Input: part model. Units: mm. Frame: model coordinates. A direction names the side the tool comes from. Give positions to 0.01 mm unless a question says otherwise; leave off trailing zeros. Loops run counter-clockwise (first coordinate to the right, second up) from the corner with the lowest first, then second, coordinate; pieces in that order, holes last. Notation, with made-up numbers: (-37, 35) - (-21, 35) arc R35 cw to (-21, 72) - close; hole circle Ø3 at (8, 47.5). An arc over 180 degrees is marked (long way). One line per item, written item: value.
from build123d import *

# Parameters (mm, degrees)
F0_W     = 40
F0_H     = 16
F1_DEPTH = 9.6
F2_R     = 2.4
F3_DEPTH = 1.8
F4_T     = -1.8


with BuildPart() as f1:
    # F0 (on Top) → F1 (new body)
    with BuildSketch(Plane.XY):
        with Locations((-20, 8)):
            Rectangle(F0_W, F0_H)
    extrude(amount=F1_DEPTH)

    # F2 (on face) → F3 (join)
    with BuildSketch(Plane.XY.offset(9.6)):
        with Locations((-36, 12)):
            Circle(F2_R)
        with Locations((-36, 4)):
            Circle(F2_R)
        with Locations((-28, 4)):
            Circle(F2_R)
        with Locations((-28, 12)):
            Circle(F2_R)
        with Locations((-20, 4)):
            Circle(F2_R)
        with Locations((-12, 4)):
            Circle(F2_R)
        with Locations((-4, 4)):
            Circle(F2_R)
        with Locations((-4, 12)):
            Circle(F2_R)
        with Locations((-12, 12)):
            Circle(F2_R)
        with Locations((-20, 12)):
            Circle(F2_R)
    extrude(amount=F3_DEPTH)

    # F4
    f4_openings = [f1.faces().sort_by_distance(p)[0] for p in [
        (-20, 8, 0),
    ]]
    offset(amount=F4_T, openings=f4_openings, kind=Kind.INTERSECTION)


solid = f1.part
Item 1: Draft query along X for faces 4 (the face through (-4, 4, 11.4)), 5 (the face through (-4.44, 4.41, 8.69)), 6 (the face through (0, 8, 5)). Return one class per face: pulls with the +X half, pulls with the -X half, needs draft (parallel to the pull), parting line crosses it, or undercut.
Verdict:
face 4: needs draft
face 5: undercut
face 6: pulls with the +X half
Item 2: Section A-A, the plane z = 4.25. Output: boundary loops of the cut face in (x, y), and give its area (3 significant figures).
Verdict:
outline: (-40, 0) - (0, 0) - (0, 16) - (-40, 16) - close; hole (-38.2, 1.8) - (-1.8, 1.8) - (-1.8, 14.2) - (-38.2, 14.2) - close
area: 189 mm^2
Item 3: Section C-C, the plane x = -12. Output: boundary loops of the cut face in (y, z), and give its area (3 significant figures).
Verdict:
outline: (0, 0) - (1.8, 0) - (1.8, 7.8) - (3.4, 7.8) - (3.4, 9.6) - (4.6, 9.6) - (4.6, 7.8) - (11.4, 7.8) - (11.4, 9.6) - (12.6, 9.6) - (12.6, 7.8) - (14.2, 7.8) - (14.2, 0) - (16, 0) - (16, 9.6) - (14.4, 9.6) - (14.4, 11.4) - (9.6, 11.4) - (9.6, 9.6) - (6.4, 9.6) - (6.4, 11.4) - (1.6, 11.4) - (1.6, 9.6) - (0, 9.6) - close
area: 69.8 mm^2
Item 4: Section D-D, the plane z = 8.5. Count the separate pieces of the cut face and the enclosed holes in it, and give its area (3 significant figures).
Verdict:
separate pieces: 1
enclosed holes: 10
area: 629 mm^2
Item 5: Material intervals for L1, parallel to Y at x = -36, z = 9.2; L2, parallel to X at y = 14, z = 0.5; L3, parallel to X at y = 12, z = 8.75, sorted ascending.
Verdict:
L1: y = 0 to 3.4, 4.6 to 11.4, 12.6 to 16
L2: x = -40 to -38.2, -1.8 to 0
L3: x = -40 to -36.6, -35.4 to -28.6, -27.4 to -20.6, -19.4 to -12.6, -11.4 to -4.6, -3.4 to 0
Item 6: Pin query (flat end, axial travel): P1, Ø0.6, axis at x = -12, y = 12, coming from the -Z side; P2, Ø1.5, axis at x = -26.5, y = 8.5, coming from the -Z side. Return the tip coordinate at first contact, or that it passes through.
Verdict:
P1: stops at z = 9.6
P2: stops at z = 7.8
Item 7: Access query for faces 1 (the face through (-20, 8, 7.8)), 2 (the face through (-38.398, 12.106, 10.487)), 3 (the face through (-36, 12, 11.4)). Directions: +Z, -Z, +X, -X, +Y, -Y. A direction counts if a zero-diameter tool reaches every point of the face in a straight line with its end or side. Return the directions, or none.
Verdict:
face 1: -Z
face 2: +Z
face 3: +Z, +X, -X, +Y, -Y
Item 8: Section B-B, the plane y = 9. Output: boundary loops of the cut face in (x, z), and give its area (3 significant figures).
Verdict:
outline: (-40, 0) - (-38.2, 0) - (-38.2, 7.8) - (-1.8, 7.8) - (-1.8, 0) - (0, 0) - (0, 9.6) - (-40, 9.6) - close
area: 100 mm^2
